The listing builds one solid part. Answer for the finished solid, in the listing's coordinates (mm). A direction names the side the tool comes from. Give positions to 0.01 mm unless a question says otherwise; leave off trailing zeros. Order: outer loops, then holes, each group sorted by start corner. A loop starts at its lowest first (then second) coordinate and runs counter-clockwise, first axis right, second up. Notation, with made-up numbers: (51, 72) - (81, 72) arc R27 ccw to (81, 92) - close; hole circle Ø11 at (61, 14.25). An arc over 180 degrees is marked (long way). Answer in a Markdown table with one row per item.
from build123d import *

# Parameters (mm, degrees)
SKETCH1_W           = 50.8
SKETCH1_H           = 38.1
BOSS_EXTRUDE1_DEPTH = 3.175
SKETCH2_W           = 4.7625
SKETCH2_H           = 38.1
BOSS_EXTRUDE2_DEPTH = 63.5
FILLET1_R           = 6.35
CUT_EXTRUDE1_REACH  = 52.8
SKETCH3_R           = 2.159
SKETCH3_W           = 20.574
SKETCH3_H           = 41.148
CUT_EXTRUDE2_REACH  = 5.175
SKETCH4_R           = 2.159
CUT_EXTRUDE3_REACH  = 52.8
SKETCH5_R           = 5.08


with BuildPart() as part:
    # Sketch1 → Boss-Extrude1 (new body)
    with BuildSketch(Plane(origin=(0, 0, 0), x_dir=(1, 0, 0), z_dir=(0, 1, 0))):
        with Locations((25.4, 19.05)):
            Rectangle(SKETCH1_W, SKETCH1_H)
    extrude(amount=BOSS_EXTRUDE1_DEPTH)

    # Sketch2 → Boss-Extrude2 (add)
    with BuildSketch(Plane(origin=(0, 3.175, 0), x_dir=(1, 0, 0), z_dir=(0, 1, 0))):
        with Locations((48.41875, 19.05)):
            Rectangle(SKETCH2_W, SKETCH2_H)
        with Locations((2.38125, 19.05)):
            Rectangle(SKETCH2_W, SKETCH2_H)
    extrude(amount=BOSS_EXTRUDE2_DEPTH)

    # Fillet1
    fillet1_edges = [part.edges().sort_by_distance(p)[0] for p in [
        (46.0375, 3.175, -19.05),
        (48.41875, 66.675, -38.1),
        (48.41875, 66.675, 0),
        (4.7625, 3.175, -19.05),
        (2.38125, 66.675, -38.1),
        (2.38125, 66.675, 0),
    ]]
    fillet(fillet1_edges, radius=FILLET1_R)

    # Sketch3 → Cut-Extrude1 (cut, up to next)
    with BuildSketch(Plane(origin=(50.8, 0, 0), x_dir=(0, 0, -1), z_dir=(1, 0, 0)), mode=Mode.PRIVATE) as cut_extrude1_sk1:
        with Locations((24.9555, 61.5315)):
            Circle(SKETCH3_R)
    cut_extrude1_tool1 = extrude(cut_extrude1_sk1.sketch, amount=-CUT_EXTRUDE1_REACH, mode=Mode.PRIVATE) & part.part
    add(cut_extrude1_tool1.solids().sort_by_distance((50.8, 61.5315, -24.9555))[0], mode=Mode.SUBTRACT)
    # Sketch3 → Cut-Extrude1 (cut, up to next)
    with BuildSketch(Plane(origin=(50.8, 0, 0), x_dir=(0, 0, -1), z_dir=(1, 0, 0)), mode=Mode.PRIVATE) as cut_extrude1_sk2:
        with Locations((13.1445, 61.5315)):
            Circle(SKETCH3_R)
    cut_extrude1_tool2 = extrude(cut_extrude1_sk2.sketch, amount=-CUT_EXTRUDE1_REACH, mode=Mode.PRIVATE) & part.part
    add(cut_extrude1_tool2.solids().sort_by_distance((50.8, 61.5315, -13.1445))[0], mode=Mode.SUBTRACT)
    # Sketch3 → Cut-Extrude1 (cut, up to next)
    with BuildSketch(Plane(origin=(50.8, 0, 0), x_dir=(0, 0, -1), z_dir=(1, 0, 0)), mode=Mode.PRIVATE) as cut_extrude1_sk3:
        with Locations((13.1445, 13.9065)):
            Circle(SKETCH3_R)
    cut_extrude1_tool3 = extrude(cut_extrude1_sk3.sketch, amount=-CUT_EXTRUDE1_REACH, mode=Mode.PRIVATE) & part.part
    add(cut_extrude1_tool3.solids().sort_by_distance((50.8, 13.9065, -13.1445))[0], mode=Mode.SUBTRACT)
    # Sketch3 → Cut-Extrude1 (cut, up to next)
    with BuildSketch(Plane(origin=(50.8, 0, 0), x_dir=(0, 0, -1), z_dir=(1, 0, 0)), mode=Mode.PRIVATE) as cut_extrude1_sk4:
        with Locations((24.9555, 13.9065)):
            Circle(SKETCH3_R)
    cut_extrude1_tool4 = extrude(cut_extrude1_sk4.sketch, amount=-CUT_EXTRUDE1_REACH, mode=Mode.PRIVATE) & part.part
    add(cut_extrude1_tool4.solids().sort_by_distance((50.8, 13.9065, -24.9555))[0], mode=Mode.SUBTRACT)
    # Sketch3 → Cut-Extrude1 (cut, up to next)
    with BuildSketch(Plane(origin=(50.8, 0, 0), x_dir=(0, 0, -1), z_dir=(1, 0, 0)), mode=Mode.PRIVATE) as cut_extrude1_sk5:
        with Locations((19.05, 37.719)):
            Rectangle(SKETCH3_W, SKETCH3_H)
    cut_extrude1_tool5 = extrude(cut_extrude1_sk5.sketch, amount=-CUT_EXTRUDE1_REACH, mode=Mode.PRIVATE) & part.part
    add(cut_extrude1_tool5.solids().sort_by_distance((50.8, 37.719, -19.05))[0], mode=Mode.SUBTRACT)

    # Sketch4 → Cut-Extrude2 (cut, up to next)
    with BuildSketch(Plane(origin=(0, 3.175, 0), x_dir=(1, 0, 0), z_dir=(0, 1, 0)), mode=Mode.PRIVATE) as cut_extrude2_sk1:
        with Locations((25.4, 28.575)):
            Circle(SKETCH4_R)
    cut_extrude2_tool1 = extrude(cut_extrude2_sk1.sketch, amount=-CUT_EXTRUDE2_REACH, mode=Mode.PRIVATE) & part.part
    add(cut_extrude2_tool1.solids().sort_by_distance((25.4, 3.175, -28.575))[0], mode=Mode.SUBTRACT)
    # Sketch4 → Cut-Extrude2 (cut, up to next)
    with BuildSketch(Plane(origin=(0, 3.175, 0), x_dir=(1, 0, 0), z_dir=(0, 1, 0)), mode=Mode.PRIVATE) as cut_extrude2_sk2:
        with Locations((25.4, 9.525)):
            Circle(SKETCH4_R)
    cut_extrude2_tool2 = extrude(cut_extrude2_sk2.sketch, amount=-CUT_EXTRUDE2_REACH, mode=Mode.PRIVATE) & part.part
    add(cut_extrude2_tool2.solids().sort_by_distance((25.4, 3.175, -9.525))[0], mode=Mode.SUBTRACT)

    # Sketch5 → Cut-Extrude3 (cut, up to next)
    with BuildSketch(Plane.ZY, mode=Mode.PRIVATE) as cut_extrude3_sk1:
        with Locations((-19.05, 47.625)):
            Circle(SKETCH5_R)
    cut_extrude3_tool1 = extrude(cut_extrude3_sk1.sketch, amount=-CUT_EXTRUDE3_REACH, mode=Mode.PRIVATE) & part.part
    add(cut_extrude3_tool1.solids().sort_by_distance((0, 47.625, -19.05))[0], mode=Mode.SUBTRACT)


solid = part.part
Item 1: Determine the mould class of faces 4 (the face through (48, 37, -8.763)), 5 (the face through (0, 33, -19)), 6 (the face through (48.452, 64.864, -36.19)), 7 (the face through (48, 37, -29.337)) for opening direction Z: pulls with the +Z half, pulls with the -Z half, needs draft (parallel to the pull), parting line crosses it, or undercut.
Answer block:
| item | result |
|---|---|
| face 4 | undercut |
| face 5 | needs draft |
| face 6 | pulls with the -Z half |
| face 7 | undercut |
Item 2: Each of these flat-tipped pins is pushed along its axis until it touches: P1, Ø7, axis at y = 61.53, z = -24.96, coming from the +X side; P2, Ø2.5, axis at y = 13.91, z = -13.14, coming from the +X side; P3, Ø9, axis at y = 47.625, z = -19.05, coming from the -X side; P4, Ø2, axis at x = 44.5, z = -14.5, coming from the +Y side. Where does it stop, or does it pass through?
Answer block:
| item | result |
|---|---|
| P1 | x = 50.8 |
| P2 | x = 4.76 |
| P3 | through |
| P4 | y = 6.97 |
Item 3: Find section A-A on z = -19.05. Count the separate pieces of the cut face and the enclosed holes in it, then the cut area to 3 significant figures.
Answer block:
| item | result |
|---|---|
| separate pieces | 3 |
| enclosed holes | 0 |
| area | 539 mm² |
Item 4: Consider line 1 (X direction, y = 26.5, z = -32.5); line 2 (Y direction, x = 2, z = -19) (3 decimals); line 3 (Y direction, x = 14, z = -35) (3 decimals). Determine where each line is inside the solid, lowest interval first.
Answer block:
| item | result |
|---|---|
| line 1 | 0 to 4.76, 46.04 to 50.8 |
| line 2 | 0 to 42.545, 52.705 to 66.675 |
| line 3 | 0 to 3.175 |
Item 5: Find section B-B on x = 25.4. Write down the section's boundary in (y, z) (3 decimals), then the cut area to 3 significant figures.
Answer block:
| item | result |
|---|---|
| outline | (0, -38.1) - (3.175, -38.1) - (3.175, -30.734) - (0, -30.734) - close; (0, -26.416) - (3.175, -26.416) - (3.175, -11.684) - (0, -11.684) - close; (0, -7.366) - (3.175, -7.366) - (3.175, 0) - (0, 0) - close |
| area | 93.5 mm² |
Item 6: Find section C-C on y = 32. Write down the section's boundary in (x, z), then the cut area to 3 significant figures.
Answer block:
| item | result |
|---|---|
| outline | (0, -38.1) - (4.76, -38.1) - (4.76, 0) - (0, 0) - close; (46.04, -38.1) - (50.8, -38.1) - (50.8, -29.34) - (46.04, -29.34) - close; (46.04, -8.76) - (50.8, -8.76) - (50.8, 0) - (46.04, 0) - close |
| area | 265 mm² |
Item 7: Find section D-D on y = 51. Write down the section's boundary in (x, z).
Answer block:
| item | result |
|---|---|
| outline | (0, -38.1) - (4.76, -38.1) - (4.76, -22.85) - (0, -22.85) - close; (0, -15.25) - (4.76, -15.25) - (4.76, 0) - (0, 0) - close; (46.04, -38.1) - (50.8, -38.1) - (50.8, -29.34) - (46.04, -29.34) - close; (46.04, -8.76) - (50.8, -8.76) - (50.8, 0) - (46.04, 0) - close |
Item 8: Which of the six approach directions +Z, -Z, +X, -X, +Y, -Y give full straight-line access (tool end or side, diameter ignored) to faces 1 (the face through (44.227, 5.085, -19.317)), 2 (the face through (48.45, 11.8, -24.49)), 3 (the face through (2.415, 64.864, -1.91))?
Answer block:
| item | result |
|---|---|
| face 1 | +Z, -Z, +Y |
| face 2 | +X |
| face 3 | +Z, +X, -X, +Y |
